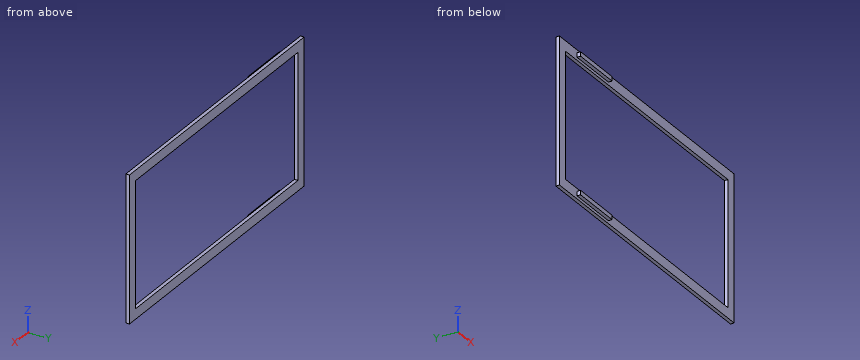
```python
from build123d import *

# Parameters (mm, degrees)
F0_W     = 2000
F0_H     = 1000
F0_W_2   = 1860
F0_H_2   = 860
F1_DEPTH = 25
F2_W     = 360
F2_H     = 30
F3_DEPTH = 25


with BuildPart() as f1:
    # F0 (on Front) → F1 (new body)
    with BuildSketch(Plane.XZ):
        with Locations((1000, -500)):
            Rectangle(F0_W, F0_H)
        with Locations((1000, -500)):
            Rectangle(F0_W_2, F0_H_2, mode=Mode.SUBTRACT)
    extrude(amount=F1_DEPTH)

    # F2 (on face) → F3 (join)
    with BuildSketch(Plane.XZ.offset(25)):
        with Locations((380, -35)):
            Rectangle(F2_W, F2_H)
        with Locations((380, -965)):
            Rectangle(F2_W, F2_H)
    extrude(amount=F3_DEPTH)


solid = f1.part
```
Source: CAD feature listing. Evaluate the final solid. Frame: model axes, mm. Coordinates: 2 decimals unless noted, no trailing zeros. Write each loop counter-clockwise with the first axis right and the second up, starting at its lowest first coordinate (ties: lowest second). Pieces come first, ordered by that corner, then holes. Notation, with made-up numbers: (-36.75, 26) - (-15.75, 26) arc R17 cw to (-15.75, 46) - close; hole circle Ø1 at (30, 76). An arc over 180 degrees is marked (long way). Answer as a JSON object with one key per item and string values.
Q1. Section query B-B, the plane z = -833. Output: boundary loops of the cut face in (x, y), plus the area to 3 significant figures.
Ans:
{"outline": "(0, -25) - (70, -25) - (70, 0) - (0, 0) - close; (1930, -25) - (2000, -25) - (2000, 0) - (1930, 0) - close", "area": "3,500 mm2"}
Q2. First-contact query: pin 1 Ø12.5 at (y, z) = (-33, -42.5) entering from +X; pin 2 Ø12.5 at (x, y) = (384, -37.5) entering from -Z; pin 3 Ø7.5 at (x, y) = (359.5, -41) entering from +Z. Flat tips, straight axial feed; report the tip coordinate or a pass-through.
Ans:
{"pin 1": "stops at x = 560", "pin 2": "stops at z = -980", "pin 3": "stops at z = -20"}
Q3. Section query A-A, the plane x = 637.5. Output: boundary loops of the cut face in (y, z), plus the area to 3 significant figures.
Ans:
{"outline": "(-25, -1000) - (0, -1000) - (0, -930) - (-25, -930) - close; (-25, -70) - (0, -70) - (0, 0) - (-25, 0) - close", "area": "3,500 mm2"}
Q4. Section query C-C, the plane y = -14.5. Output: boundary loops of the cut face in (x, z), plus the area to 3 significant figures.
Ans:
{"outline": "(0, -1000) - (2000, -1000) - (2000, 0) - (0, 0) - close; hole (70, -930) - (1930, -930) - (1930, -70) - (70, -70) - close", "area": "400,000 mm2"}
Q5. Material intervals for line 1 (Z direction, x = 1280, y = -22.5); line 2 (X direction, y = -5.5, z = -780.5); line 3 (Y direction, x = 1421.5, z = -59.5), sorted ascending. Write a range as [from, to].
Ans:
{"line 1": "z = [-1000, -930], [-70, 0]", "line 2": "x = [0, 70], [1930, 2000]", "line 3": "y = [-25, 0]"}
